Verification items for the finished model (mm, model axes). A direction names the side the tool comes from. Coordinates: 2 decimals unless noted, no trailing zeros. Order: outer loops, then holes, each group sorted by start corner. A loop starts at its lowest first (then second) coordinate and runs counter-clockwise, first axis right, second up.
Q1. Cross-section at B-B, the plane x = -29. Record the boundary of the cut face in (y, z).
Q2. Set-up check for faces 4 (the flat face through (29.4, 30, 29.4)), 5 (the flat face through (24, 16, 2)), 6 (the flat face through (-17, 0, -17)), 7 (the flat face through (25, 15, 0)): record each of +Z, -Z, +X, -X, +Y, -Y from which the full face is reachable in a straight line by a thin tool's end or side.
Q3. Thickness scan on line 1 (X direction, y = 10, z = -0.5); line 2 (Z direction, x = 2, y = -1); line 3 (X direction, y = 3, z = -22). Record the ranges inside material, lowest first.
Q4. Cross-section at A-A, the plane y = 10. Record the boundary of the cut face in (x, z), and give its area (3 significant figures).
Q5. Cross-section at C-C, the plane z = 13. Record the boundary of the cut face in (x, y).
Q6. Depth check by flat-ended pin: P1, Ø0.6, axis at y = 15.5, z = -0.5, coming from the -X side; P2, Ø3, axis at x = 2.5, y = 10, coming from the +Z side; P3, Ø14, axis at x = 18, y = 13, coming from the +Z side. Enter the tip coordinate at first touch or a pass-through.
Q7. Draft check along X on faces 1 (the flat face through (0, 15, -25)), 2 (the flat face through (-33, 30, -25)), 3 (the cylindrical face through (28.69, 15.8, 29.29)). Enter one of: pulls with the +X half, pulls with the -X half, needs draft (parallel to the pull), parting line crosses it, or undercut.
from build123d import *
from build123d.topology import SkipClean

# Parameters (mm, degrees)
EXTRUDE_1_DEPTH      = 30
CUT_EXTRUDE_1_DEPTH  = 68.808554033
SHELL_START          = 2
SHELL_1_DEPTH        = 28
EXTRUDE_2_DEPTH      = 4.5
EXTRUDE_2_DEPTH_BACK = 34.5
SKETCH_3_R           = 7


# Read off the part's stored shape, not the designer's step: 抽壳1
with BuildPart() as part:
    # 草图1 → 凸台-拉伸1 (new body)
    with BuildSketch(Plane(origin=(0, 0, 0), x_dir=(1, 0, 0), z_dir=(0, 1, 0))):
        with BuildLine():
            Line((0, 7), (0, 43))
            ThreePointArc((0, 43), (-30.405591591, 30.405591591), (-43, 0))
            Line((-43, 0), (-7, 0))
            ThreePointArc((-7, 0), (-4.949747468, -4.949747468), (0, -7))
            Line((0, -7), (0, -43))
            ThreePointArc((0, -43), (30.405591591, -30.405591591), (43, 0))
            Line((43, 0), (7, 0))
            ThreePointArc((7, 0), (4.949747468, 4.949747468), (0, 7))
        make_face()
    extrude(amount=EXTRUDE_1_DEPTH)

    # 草图2 → 切除-拉伸1 (cut, through all)
    with BuildSketch(Plane(origin=(0, 30, 0), x_dir=(1, 0, 0), z_dir=(0, 1, 0))):
        Polygon((1, -1), (1, -3.5), (-1, -3.5), (-1, -1), (-3.5, -1), (-3.5, 1), (-1, 1), (-1, 3.5), (1, 3.5), (1, 1), (3.5, 1), (3.5, -1), align=None)
    extrude(amount=-CUT_EXTRUDE_1_DEPTH, mode=Mode.SUBTRACT)

    # 抽壳1 outline → 抽壳1 (cut)
    with BuildSketch(Plane(origin=(0, 0, 0), x_dir=(1, 0, 0), z_dir=(0, 1, 0)).offset(SHELL_START)):
        with BuildLine():
            Line((3, -3), (3, -5.5))
            Line((3, -5.5), (2, -5.5))
            Line((2, -5.5), (2, -40.951190459))
            ThreePointArc((2, -40.951190459), (28.991378029, -28.991378029), (40.951190459, -2))
            Line((40.951190459, -2), (5.5, -2))
            Line((5.5, -2), (5.5, -3))
            Line((5.5, -3), (3, -3))
        make_face()
        with BuildLine():
            Line((3, 4), (3, 3))
            Line((3, 3), (4, 3))
            ThreePointArc((4, 3), (3.535533906, 3.535533906), (3, 4))
        make_face()
        with BuildLine():
            Line((-3, -3), (-4, -3))
            ThreePointArc((-4, -3), (-3.535533906, -3.535533906), (-3, -4))
            Line((-3, -4), (-3, -3))
        make_face()
        with BuildLine():
            ThreePointArc((-2, 40.951190459), (-28.991378029, 28.991378029), (-40.951190459, 2))
            Line((-40.951190459, 2), (-5.5, 2))
            Line((-5.5, 2), (-5.5, 3))
            Line((-5.5, 3), (-3, 3))
            Line((-3, 3), (-3, 5.5))
            Line((-3, 5.5), (-2, 5.5))
            Line((-2, 5.5), (-2, 40.951190459))
        make_face()
    extrude(amount=SHELL_1_DEPTH, mode=Mode.SUBTRACT)

    # 草图3 → 凸台-拉伸2 (add, two sides: drawn at the far end of the back side and taken through both)
    with SkipClean():  # the faces are left unmerged after this step: merging them gives an invalid solid
        with BuildSketch(Plane(origin=(0, 30, 0), x_dir=(1, 0, 0), z_dir=(0, 1, 0)).offset(-EXTRUDE_2_DEPTH_BACK)):
            with Locations(Location((0, 0, 0), (0, 0, 270))):
                Circle(SKETCH_3_R)
            Polygon((-3.5, 1), (-1, 1), (-1, 3.5), (1, 3.5), (1, 1), (3.5, 1), (3.5, -1), (1, -1), (1, -3.5), (-1, -3.5), (-1, -1), (-3.5, -1), align=None, mode=Mode.SUBTRACT)
        extrude(amount=EXTRUDE_2_DEPTH + EXTRUDE_2_DEPTH_BACK)


solid = part.part
Check values:
1. outline: (0, -31.75) - (30, -31.75) - (30, -28.98) - (2, -28.98) - (2, -2) - (30, -2) - (30, 0) - (0, 0) - close
2. face 4: +Z, +X, +Y
2. face 5: +Y
2. face 6: -Z, -X, -Y
2. face 7: -Z, +X, +Y, -Y
3. line 1: x = -43 to -3.5, 3.5 to 6.98
3. line 2: z = -6.71 to -1, 1 to 6.71
3. line 3: x = -36.95 to -34.6, -2 to 0
4. outline: (-43, 0) arc R43 ccw to (0, -43) - (0, -7) arc R7 ccw to (7, 0) - (43, 0) arc R43 ccw to (0, 43) - (0, 7) arc R7 ccw to (-7, 0) - close; hole (-40.95, -2) arc R41 ccw to (-2, -40.95) - (-2, -6.71) arc R7 cw to (-6.71, -2) - close; hole (-3.5, -1) - (-1, -1) - (-1, -3.5) - (1, -3.5) - (1, -1) - (3.5, -1) - (3.5, 1) - (1, 1) - (1, 3.5) - (-1, 3.5) - (-1, 1) - (-3.5, 1) - close; hole (2, 6.71) arc R7 cw to (6.71, 2) - (40.95, 2) arc R41 ccw to (2, 40.95) - close
4. area: 666 mm2
5. outline: (0, 0) - (40.99, 0) - (40.99, 30) - (38.88, 30) - (38.88, 2) - (2, 2) - (2, 30) - (0, 30) - close
6. P1: stops at x = -43
6. P2: stops at z = 42.99
6. P3: stops at z = 41.57
7. face 1: pulls with the +X half
7. face 2: needs draft
7. face 3: undercut
